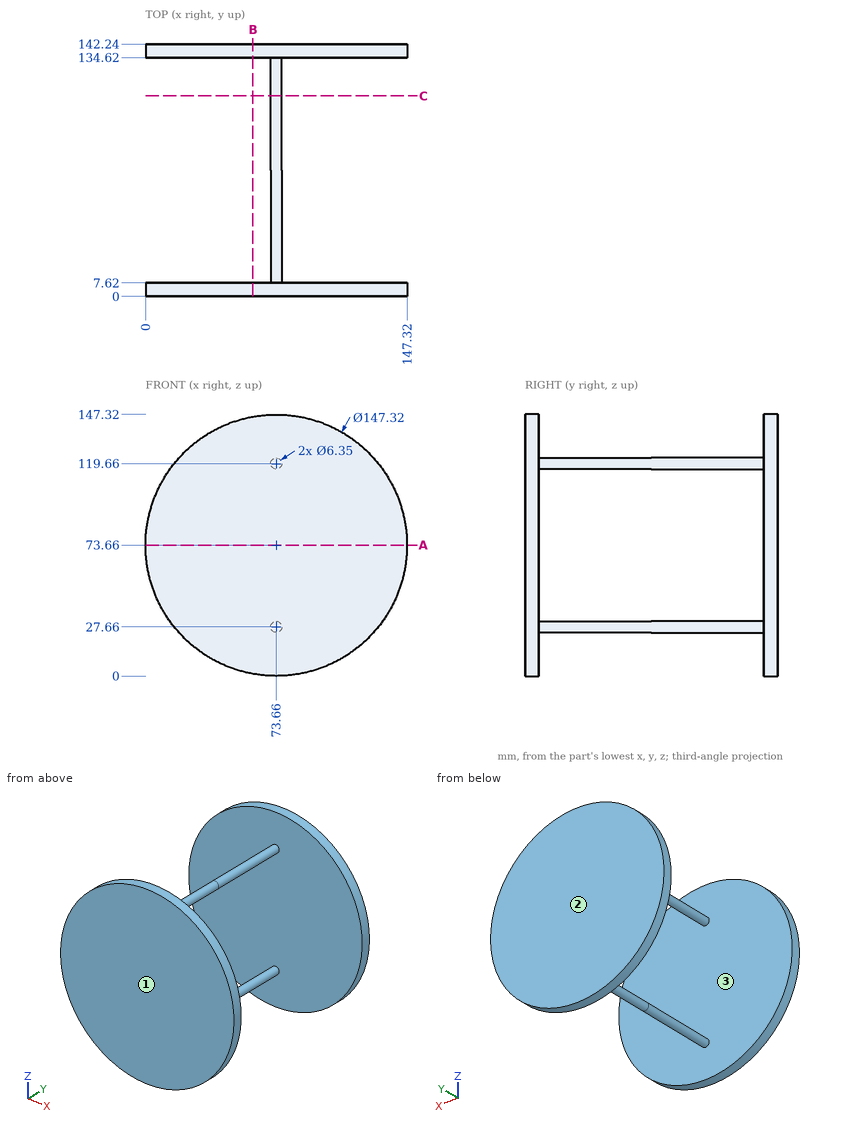
Drawing for the job (mm, zero at the part's lowest x, y, z). Round coordinates to 2 decimals unless told otherwise and drop trailing zeros. Order: outer loops, then holes, each group sorted by start corner. A loop starts at its lowest first (then second) coordinate and runs counter-clockwise, first axis right, second up.
Item 1: Saw through at A-A on z = 73.66. Write the cut outline in (x, y).
Item 2: Saw through at B-B on x = 60.5. Write the cut outline in (y, z).
Item 3: Probe line 1 along Y through (x, z) = (120, 42.5); line 2 along Z through (x, y) = (72.5, 10.5); line 3 along X through (y, z) = (71, 119). List the from-to ranges inside material, lowest first.
Item 4: Mould opens along Y. For the marked faces 1, 2 and 3 say: pulls with the +Y half, pulls with the -Y half, needs draft (parallel to the pull), parting line crosses it, or undercut.
Item 5: Saw through at C-C on y = 113. Write the cut outline in (x, z) (3 decimals).
Item 6: Pin check, flat tip, straight feed: pin 1 (10 mm diameter, centred on x = 68.5, y = 21, fed in from -Z). Stop position of the tip, or through.
Reported:
1. outline: (0, 0) - (147.32, 0) - (147.32, 7.62) - (0, 7.62) - close; (0, 134.62) - (147.32, 134.62) - (147.32, 142.24) - (0, 142.24) - close
2. outline: (0, 1.19) - (7.62, 1.19) - (7.62, 146.13) - (0, 146.13) - close; (134.62, 1.19) - (142.24, 1.19) - (142.24, 146.13) - (134.62, 146.13) - close
3. line 1: y = 0 to 7.62, 134.62 to 142.24
3. line 2: z = 24.7 to 30.62, 116.7 to 122.62
3. line 3: x = 70.55 to 76.77
4. face 1: pulls with the -Y half
4. face 2: pulls with the +Y half
4. face 3: undercut
5. outline: circle Ø6.35 at (73.66, 27.66); circle Ø6.35 at (73.66, 119.66)
6. pin 1: stops at z = 24.49
